The drawing under review shows one solid part. Ordinate dimensions are in mm from its lowest x, y, z. A direction names the side the tool comes from. Give positions to 0.01 mm unless a question says otherwise; leave off trailing zeros. Order: outer loops, then holes, each group sorted by start corner. A loop starts at its lowest first (then second) coordinate and runs counter-clockwise, first axis right, second up. Notation, with made-up numbers: M 34,-36 L 89,-36 A10 cw 89,-23 Z; hole C 35,-34.5 d9. An arc over 180 degrees is marked long. Put each result on its own line as item: value. Start each with the question number.
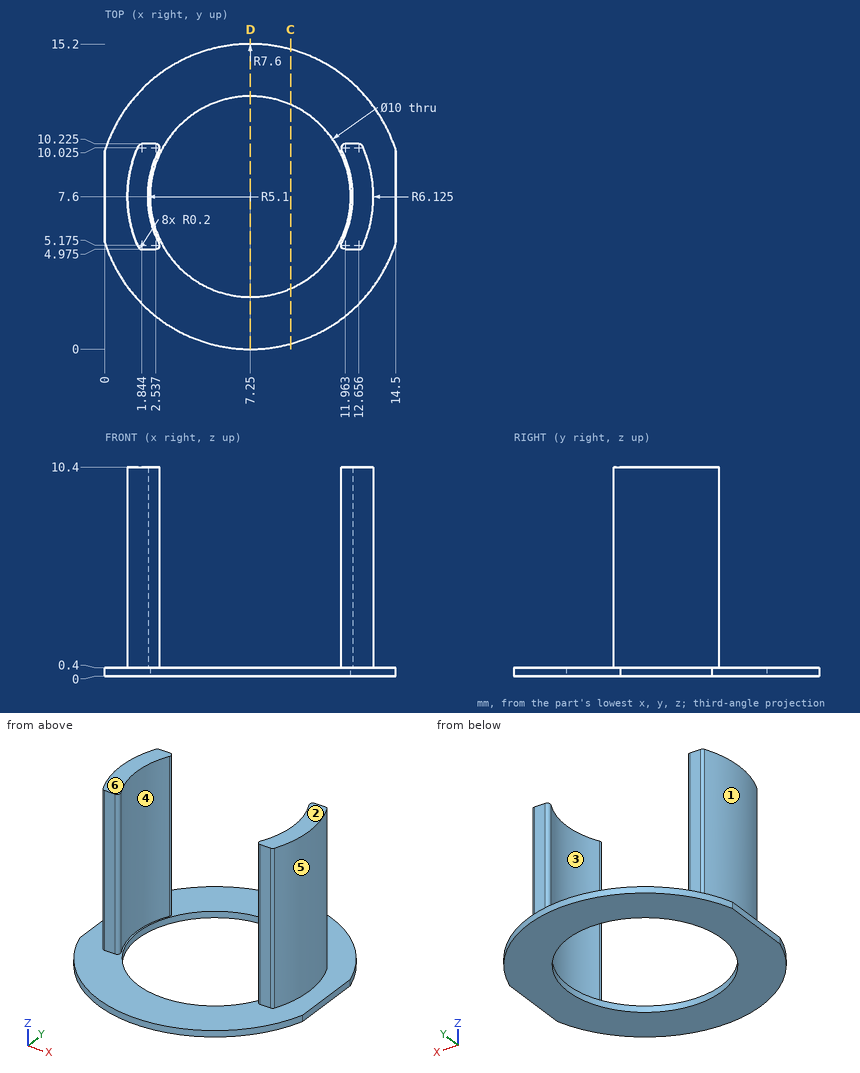
1. Consider section C-C on x = 9.25. Give the boundary of the cut face in (y, z).
2. Insertion check: pin 1 (2 mm diameter, centred on x = 3, z = 3.5, fed in from +Y) (3 decimals); pin 2 (2 mm diameter, centred on y = 6, z = 7, fed in from +X); pin 3 (0.6 mm diameter, centred on x = 2.5, z = 4.5, fed in from -Y) (3 decimals). Each pin has a flat end and moves straight along its axis. Give the tip position at first contact, or say it passes through.
3. Consider section D-D on x = 7.25. Give the boundary of the cut face in (y, z).
4. The part is to be moulded in two halves that separate along Y. For the marked faces 1, 2 and 3, say which applies: +Y half, -Y half, draft (parallel to the pull), parting line (faces both ways), or undercut.
5. To check wall thickness, follow probe 1 along Y at (x, z) = (7.25, 0.1); probe 2 along Z at (x, y) = (12, 11.75); probe 3 along Y at (x, z) = (2, 7.25) (1 decimal). State the ranges of each line that lie inside material, in increasing order.
6. Machinability: for the marked faces 4, 5 and 6, which of the approach directions +Z, -Z, +X, -X, +Y, -Y give a long, thin tool a straight path to every point of the face, cutting with its end or side? Answer none if there is none.
Returned:
1. outline: M 0.27,0 L 3.02,0 L 3.02,0.4 L 0.27,0.4 Z; M 12.18,0 L 14.93,0 L 14.93,0.4 L 12.18,0.4 Z
2. pin 1: stops at y = 10.225
2. pin 2: stops at x = 13.35
2. pin 3: stops at y = 4.975
3. outline: M 0,0 L 2.6,0 L 2.6,0.4 L 0,0.4 Z; M 12.6,0 L 15.2,0 L 15.2,0.4 L 12.6,0.4 Z
4. face 1: parting line
4. face 2: draft
4. face 3: undercut
5. probe 1: y = 0 to 2.6, 12.6 to 15.2
5. probe 2: z = 0 to 0.4
5. probe 3: y = 5 to 10.2
6. face 4: +Z
6. face 5: +Z, +X
6. face 6: +Z, +X, -X, +Y, -Y
